Check sheet for the modelled part. Datum: model origin and axes. Units: mm. Round coordinates to 2 decimals unless told otherwise and drop trailing zeros. Order: outer loops, then holes, each group sorted by start corner. A loop starts at its lowest first (then second) coordinate and runs counter-clockwise, first axis right, second up. Notation, with made-up numbers: (76, 53.5) -> (123, 53.5) arc R19 ccw to (123, 86.5) -> close; hole circle Ø1 at (-36, -29). An arc over 180 degrees is marked (long way). Answer in a Markdown table with one row per item. Add a question column.
1. Sectioned sample at C-C, the plane x = -62.5. Record the boundary of the cut face in (y, z) (3 decimals), then the cut area to 3 significant figures.
2. Draft check along Y on faces 1 (the flat face through (-26, -63.5, 7)), 2 (the flat face through (0, -1, 7)), 3 (the cylindrical face through (-80.4, 0.3, 6.6)). Enter one of: +Y half, -Y half, draft (parallel to the pull), parting line (faces both ways), or undercut.
3. Sectioned sample at A-A, the plane z = -293.5. Record the boundary of the cut face in (x, y).
4. Material ranges on L1, parallel to Z at x = -9, y = 0 (3 decimals); L2, parallel to X at y = 40.5, z = -182; L3, parallel to X at y = -31, z = -46, recorded low to high. Write a range as from..to.
5. Depth check by flat-ended pin: P1, Ø5, axis at y = 45, z = -230, coming from the -X side; P2, Ø6.5, axis at y = 0, z = -171.577, coming from the +X side; P3, Ø7.5, axis at y = 0, z = 171.323, coming from the -X side. Enter the tip coordinate at first touch or a pass-through.
6. Sectioned sample at B-B, the plane y = 42. Record the boundary of the cut face in (x, z) (3 decimals), then the cut area to 3 significant figures.
```python
from build123d import *

# Parameters (mm, degrees)
EXTRUDE1_DEPTH               = 473.075
A_0_234_DIAMETER_HOLE1_D     = 8.128
A_0_234_DIAMETER_HOLE1_DEPTH = 19.05
A_0_234_DIAMETER_HOLE1_TIP   = 2.441897556


with BuildPart() as part:
    # Sketch1 → Extrude1 (new, symmetric)
    with BuildSketch(Plane.XY):
        with BuildLine():
            Line((-81.45600692, -19.8133218), (-82.370570719, -28.379308014))
            ThreePointArc((-82.370570719, -28.379308014), (-74.412305802, -52.975492096), (-50.8, -63.5))
            Line((-50.8, -63.5), (0, -63.5))
            Line((0, -63.5), (0, 63.5))
            Line((0, 63.5), (-50.8, 63.5))
            ThreePointArc((-50.8, 63.5), (-74.412305802, 52.975492096), (-82.370570719, 28.379308014))
            Line((-82.370570719, 28.379308014), (-81.45600692, 19.8133218))
            ThreePointArc((-81.45600692, 19.8133218), (-80.401300618, 0), (-81.45600692, -19.8133218))
        make_face()
    extrude(amount=EXTRUDE1_DEPTH, both=True)

    # A (0.234) Diameter Hole1
    with Locations(Plane(origin=(0, 0, 171.323), x_dir=(0, 1, 0), z_dir=(1, 0, 0))):
        with Locations((0, 0), (0, -342.9)):
            Hole(A_0_234_DIAMETER_HOLE1_D / 2, depth=A_0_234_DIAMETER_HOLE1_DEPTH)
            with Locations((0, 0, -(A_0_234_DIAMETER_HOLE1_DEPTH + A_0_234_DIAMETER_HOLE1_TIP / 2))):  # 118° drill point
                Cone(0, A_0_234_DIAMETER_HOLE1_D / 2, A_0_234_DIAMETER_HOLE1_TIP, mode=Mode.SUBTRACT)


solid = part.part
```
Answer key:
| question | item | result |
|---|---|---|
| 1 | outline | (-61.266, -473.075) -> (61.266, -473.075) -> (61.266, 473.075) -> (-61.266, 473.075) -> close |
| 1 | area | 116,000 mm² |
| 2 | face 1 | -Y half |
| 2 | face 2 | draft |
| 2 | face 3 | undercut |
| 3 | outline | (-82.37, -28.38) arc R31.75 ccw to (-50.8, -63.5) -> (0, -63.5) -> (0, 63.5) -> (-50.8, 63.5) arc R31.75 ccw to (-82.37, 28.38) -> (-81.46, 19.81) arc R186.63 cw to (-81.46, -19.81) -> close |
| 4 | L1 | z = -473.075..-175.641, -167.513..167.259, 175.387..473.075 |
| 4 | L2 | x = -81.32..0 |
| 4 | L3 | x = -82.54..0 |
| 5 | P1 | stops at x = -80.67 |
| 5 | P2 | stops at x = -19.54 |
| 5 | P3 | stops at x = -80.44 |
| 6 | outline | (-80.85, -473.075) -> (0, -473.075) -> (0, 473.075) -> (-80.85, 473.075) -> close |
| 6 | area | 76,500 mm² |
